Read the model definition and answer for the solid it produces. Units are mm, in the model's axes. Face numbers are marked on the shaded views. A direction names the side the tool comes from. Give positions to 0.01 mm unless a question says otherwise; leave off trailing zeros. Order: outer loops, then holes, each group sorted by start corner. A loop starts at its lowest first (then second) coordinate and runs counter-clockwise, first axis right, second up.
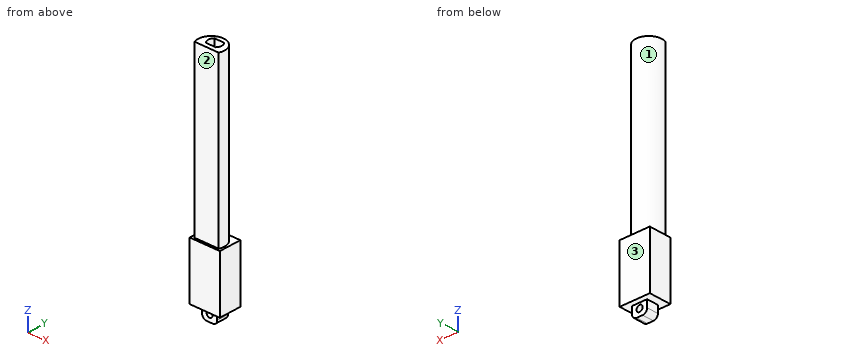
Autodesk Inventor part; units mm, degrees
ref_plane "YZ Plane" through (0, 0, 0) normal (1, 0, 0) x (0, 1, 0)
ref_plane "XZ Plane" through (0, 0, 0) normal (0, 1, 0) x (-1, 0, 0)
ref_plane "XY Plane" through (0, 0, 0) normal (0, 0, 1) x (1, 0, 0)
sketch "Sketch1" plane through (0, 0, 0) normal (0, 0, 1) x (1, 0, 0)
  line L0 (0, 0) -> (20, 0)
  line L1 (20, 0) -> (20, -14.8)
  line L2 (20, -14.8) -> (0, -14.8)
  line L3 (0, -14.8) -> (0, 0)
  dimension "d0" = 20
  dimension "d1" = 14.8
extrude "Extrusion1" add sketch "Sketch1" along normal blind 37.4
sketch "Sketch2" plane through (0, 0, 37.4) normal (0, 0, 1) x (1, 0, 0)
  line L0 (0, 0) -> (0, -14.8)
  line L1 (20, 0) -> (0, 0)
  line L2 (2, -13.4) -> (18, -13.4)
  arc A0 (18, -13.4) -> (2, -13.4) centre (10, -10.0667) ccw
  point P0 (10, -7.4)
  point P1 (10, -13.4)
extrude "Extrusion2" add sketch "Sketch2" along normal blind 120
sketch "Sketch3" plane through (0, 0, 157.4) normal (0, 0, 1) x (1, 0, 0)
  arc A0 (18, -13.4) -> (2, -13.4) centre (10, -10.0667) ccw
  line L0 (2, -13.4) -> (18, -13.4)
  line L1 (2, -13.4) -> (2, -13.4)
  line L2 (2, -13.4) -> (2, -13.4) construction
  line L3 (10, -13.4) -> (22, -13.4) construction
  line L4 (18, -13.4) -> (2, -13.4)
  line L5 (0, -14.8) -> (20, -14.8)
  line L6 (6.6913, -4.35) -> (13.3087, -4.35)
  line L7 (6.6913, -10.45) -> (13.3087, -10.45)
  arc A1 (6.6913, -4.35) -> (6.6913, -10.45) centre (10, -7.4) ccw
  arc A2 (13.3087, -10.45) -> (13.3087, -4.35) centre (10, -7.4) ccw
  point P0 (0, 0)
  dimension "d12" = 90
extrude "Extrusion3" add sketch "Sketch3" along normal blind 9.3 contours L6 A2 L7 A1
sketch "Sketch4" plane through (6.6913, -4.35, 157.4) normal (0, 1, 0) x (1, 0, 0)
  circle A0 centre (3.3087, -4.5) radius 2
  line L0 (-5.358, 0) -> (11.9754, 0)
  point P0 (-6.6913, 157.4)
  point P1 (11.3087, 0)
  point P2 (-4.6913, 0)
  dimension "d21" = 4
  dimension "d22" = 4.5
extrude "Extrusion4" cut sketch "Sketch4" against normal through all
sketch "Sketch5" plane through (0, 0, 0) normal (0, 0, -1) x (-1, 0, 0)
  line L0 (-15, -3.5) -> (-5, -3.5)
  line L1 (-5, -3.5) -> (-5, -11.3)
  line L2 (-5, -11.3) -> (-15, -11.3)
  line L3 (-15, -11.3) -> (-15, -3.5)
  line L4 (-15, -3.5) -> (-5, -11.3) construction
  line L5 (-5, -3.5) -> (-15, -11.3) construction
  line L6 (-20, 0) -> (0, 0)
  line L7 (0, -14.8) -> (-20, -14.8)
  line L8 (0, 0) -> (0, -14.8)
  line L9 (-20, 0) -> (0, 0)
  line L10 (-20, -14.8) -> (-20, 0)
  point P0 (-10, -7.4)
  point P1 (0, -7.4)
  point P2 (-10, -7.4)
  dimension "d25" = 7.8
  dimension "d26" = 10
  dimension "d27" = 10
extrude "Extrusion5" add sketch "Sketch5" along normal blind 7.8 contours L0 L1 L2 L3
sketch "Sketch6" plane through (5, -3.5, 0) normal (0, 1, 0) x (1, 0, 0)
  circle A0 centre (5, 3.3) radius 2
  line L0 (0, 7.8) -> (10, 7.8)
  line L1 (0, 0) -> (0, 7.8)
  point P0 (-5, 0)
  point P1 (5, 7.8)
  dimension "d30" = 4
  dimension "d31" = 4.5
  dimension "d32" = 5
extrude "Extrusion6" cut sketch "Sketch6" against normal through all
fillet "Fillet1" radius 3 2 edges at (15, -7.4, -7.8) (5, -7.4, -7.8)
ref_plane "작업 평면1" through (0, 0, 157.4) normal (0, 0, 1) x (1, 0, 0)
extrude "돌출7" cut sketch "Sketch3" against normal blind 100 contours L6 A2 L7 A1
split "분할1" plane through (0, 0, 157.4) removes the side toward (0, 0, 1)
sketch "스케치7" plane through (0, 0, 166.7) normal (0, 0, 1) x (1, 0, 0)
  point P0 (0, 0)
move faces "이동2" translate (0, 0, -10) faces at (8.8971, -12.4167, 157.4)
move faces "이동7" translate (0, 0, -5) faces at (11.454, -8.4605, 57.4)
properties part number "Actuator Body"
1) The part is cut by section A-A on x = 10. Determine the outline of the cut face in (y, z).
Final values:
outline: (-14.8, 0) - (-11.3, 0) - (-11.3, -1.3) - (-3.5, -1.3) - (-3.5, 0) - (0, 0) - (0, 37.4) - (-1.4, 37.4) - (-1.4, 147.4) - (-4.35, 147.4) - (-4.35, 52.4) - (-10.45, 52.4) - (-10.45, 147.4) - (-13.4, 147.4) - (-13.4, 37.4) - (-14.8, 37.4) - close; (-11.3, -7.8) - (-3.5, -7.8) - (-3.5, -5.3) - (-11.3, -5.3) - close
2) The part is cut by section C-C on y = -6. Determine the outline of the cut face in (x, z), and give its area (3 significant figures).
Final values:
outline: (0, 0) - (5, 0) - (5, -4.8) arc R3 ccw to (8, -7.8) - (12, -7.8) arc R3 ccw to (15, -4.8) - (15, 0) - (20, 0) - (20, 37.4) - (17.65, 37.4) - (17.65, 147.4) - (14.28, 147.4) - (14.28, 52.4) - (5.72, 52.4) - (5.72, 147.4) - (2.35, 147.4) - (2.35, 37.4) - (0, 37.4) - close; hole circle Ø4 at (10, -3.3)
area: 1,680 mm2
3) Given pin 1 (2.5 mm diameter, centred on x = 11.5, z = -2.5, fed in from -Y); pin 2 (5.5 mm diameter, centred on x = 9, z = 101, fed in from +Y); pin 3 (2 mm diameter, centred on x = 11, z = 56, fed in from -Y), each flat-ended and moving along its own axis, determine where each tip first touches the part or whether it passes through.
Final values:
pin 1: stops at y = -11.3
pin 2: stops at y = -1.4
pin 3: stops at y = -13.4
4) The part is cut by section D-D on z = 83. Determine the outline of the cut face in (x, y).
Final values:
outline: (2, -13.4) - (18, -13.4) arc R8.67 ccw (long way) to start; hole (6.69, -10.45) - (13.31, -10.45) arc R4.5 ccw to (13.31, -4.35) - (6.69, -4.35) arc R4.5 ccw to start
5) The part is cut by section B-B on z = -3.3. Determine the outline of the cut face in (x, y), and give its area (3 significant figures).
Final values:
outline: (5, -11.3) - (8, -11.3) - (8, -3.5) - (5, -3.5) - close; (12, -11.3) - (15, -11.3) - (15, -3.5) - (12, -3.5) - close
area: 46.8 mm2
6) Consider L1, parallel to Z at x = 10, y = -8; L2, parallel to X at y = -7.5, z = -3.3; L3, parallel to Z at x = 2.75, y = -5. Determine where each line is inside the solid, lowest interval first.
Final values:
L1: z = -7.8 to -5.3, -1.3 to 52.4
L2: x = 5 to 8, 12 to 15
L3: z = 0 to 37.4
7) A tool of negligible diameter and unlimited length cuts with its end or side. For the marked faces 1, 2 and 3, from which of +Z, -Z, +X, -X, +Y, -Y can it reach the whole face along a straight path? Write none if from no direction.
Final values:
face 1: +Z
face 2: +Z, +X, -X, -Y
face 3: +Z, -Z, +X, -X, +Y
